Autodesk Inventor part; units mm, degrees
ref_plane "Pracovní rovina2" through (5, 0, -33.5) normal (0, 0, -1) x (-1, 0, 0)
ref_plane "YZ Plane" through (0, 0, 0) normal (1, 0, 0) x (0, 1, 0)
ref_plane "XZ Plane" through (0, 0, 0) normal (0, 1, 0) x (-1, 0, 0)
sketch "Náčrt1" plane through (0, 0, 0) normal (0, 0, 1) x (1, 0, 0)
  line L0 (-11.4, 6.1) -> (11.4, 6.1)
  line L1 (11.4, 6.1) -> (11.4, -6.1)
  line L2 (11.4, -6.1) -> (-11.4, -6.1)
  line L3 (-11.4, -6.1) -> (-11.4, 6.1)
  line L4 (0, 8.54) -> (0, -8.54)
  line L5 (-15.96, 0) -> (15.96, 0)
  point P0 (0, 0)
  dimension "d0" = 22.8
  dimension "d1" = 12.2
extrude "Vysunutí1" add sketch "Náčrt1" against normal blind 28.5
ref_plane "Pracovní rovina1" through (0, 0, -17) normal (0, 0, 1) x (1, 0, 0)
sketch "Náčrt2" plane through (0, 0, -17) normal (0, 0, 1) x (1, 0, 0)
  line L0 (11.4, 6.1) -> (11.4, -6.1)
  line L1 (11.4, -6.1) -> (-11.4, -6.1)
  line L2 (-11.4, -6.1) -> (-11.4, 6.1)
  line L3 (-11.4, 6.1) -> (11.4, 6.1)
  line L4 (16.25, 6.1) -> (-16.25, 6.1)
  line L5 (-16.25, 6.1) -> (-16.25, -6.1)
  line L6 (-16.25, -6.1) -> (16.25, -6.1)
  line L7 (16.25, -6.1) -> (16.25, 6.1)
  line L8 (-22.75, 0) -> (22.75, 0)
  line L9 (0, 8.54) -> (0, -8.54)
  point P0 (0, 0)
  dimension "d5" = 32.5
  dimension "d6" = 12.2
extrude "Vysunutí2" add sketch "Náčrt2" against normal blind 2
ref_plane "Pracovní rovina2" through (5, 0, -33.5) normal (0, 0, -1) x (-1, 0, 0)
sketch "Náčrt4" plane through (5, 0, -33.5) normal (0, 0, -1) x (-1, 0, 0)
  circle A0 centre (0, 0) radius 2.5
  circle A1 centre (0, 14.2756) radius 2.5
  line L0 (2.5, 14.2756) -> (2.5, 0)
  line L1 (-26.45, 0) -> (29.2, 0)
  line L2 (5, -10.6881) -> (5, 21.4288)
  line L3 (-2.5, 14.2756) -> (-2.5, 0)
  point P0 (5, 0)
  dimension "d15" = 90
  dimension "d16" = 2.5
extrude "Vysunutí4" add sketch "Náčrt4" against normal blind 5
properties part number "Servo" material "LCP plast"
Geometry: final body of the model. Coordinates: model frame, mm. A direction names the side the tool comes from. Coordinates: 2 decimals unless noted, no trailing zeros. Order: outer loops, then holes, each group sorted by start corner. A loop starts at its lowest first (then second) coordinate and runs counter-clockwise, first axis right, second up. Notation, with made-up numbers: (17.25, 55) - (38.25, 55) arc R23 ccw to (38.25, 64) - close; hole circle Ø4 at (56, 13.25). An arc over 180 degrees is marked (long way). Return JSON: item names as keys, results as strings. Group by question number.
1. Set-up query: faces 1 (the face through (11.4, 0, -24)), 2 (the face through (14, 0, -17)), 3 (the face through (-14, 0, -19)), 4 (the face through (0, 6.1, -14)). Return all of +Z, -Z, +X, -X, +Y, -Y with unobstructed straight access to the full face (end or side cutting, diameter ignored); none if empty.
2. Cut plane B-B (x = 5). Output: boundary loops of the cut face in (y, z), plus the area to 3 significant figures.
3. Material intervals for line 1 along X through (y, z) = (-3, -28); line 2 along X through (y, z) = (14.5, -30.5); line 3 along Y through (x, z) = (-11, -13), sorted ascending. Write a range as [from, to].
4. Cut plane A-A (y = 0.5). Output: boundary loops of the cut face in (x, z), plus the area to 3 significant figures.
5. Pin query (flat end, axial travel): pin 1 (5.5 mm diameter, centred on x = -13, y = 0.5, fed in from -Z); pin 2 (8 mm diameter, centred on x = 4, y = 13.5, fed in from +Z); pin 3 (10 mm diameter, centred on y = -2, z = -11, fed in from -X); pin 4 (6 mm diameter, centred on x = 1, y = 1, fed in from -Z). Return the tip coordinate at first contact, or that it passes through.
6. Cut plane C-C (z = -18). Output: boundary loops of the cut face in (x, y).
7. Cut plane D-D (z = -26.5). Output: boundary loops of the cut face in (x, y).
Resolved:
{
 "1": {"face 1": "-Z, +X, +Y, -Y", "face 2": "+Z, +X, +Y, -Y", "face 3": "-Z, -X, +Y, -Y", "face 4": "+Z, +X, -X, +Y"},
 "2": {"outline": "(-6.1, -28.5) - (-2.5, -28.5) - (-2.5, -33.5) - (16.78, -33.5) - (16.78, -28.5) - (6.1, -28.5) - (6.1, 0) - (-6.1, 0) - close", "area": "444 mm²"},
 "3": {"line 1": "x = [-11.4, 11.4]", "line 2": "x = [2.51, 7.49]", "line 3": "y = [-6.1, 6.1]"},
 "4": {"outline": "(-16.25, -19) - (-11.4, -19) - (-11.4, -28.5) - (2.5, -28.5) - (2.5, -33.5) - (7.5, -33.5) - (7.5, -28.5) - (11.4, -28.5) - (11.4, -19) - (16.25, -19) - (16.25, -17) - (11.4, -17) - (11.4, 0) - (-11.4, 0) - (-11.4, -17) - (-16.25, -17) - close", "area": "694 mm²"},
 "5": {"pin 1": "stops at z = -28.5", "pin 2": "stops at z = -28.5", "pin 3": "stops at x = -11.4", "pin 4": "stops at z = -33.5"},
 "6": {"outline": "(-16.25, -6.1) - (16.25, -6.1) - (16.25, 6.1) - (-16.25, 6.1) - close"},
 "7": {"outline": "(-11.4, -6.1) - (11.4, -6.1) - (11.4, 6.1) - (-11.4, 6.1) - close"}
}
